Source: three-view drawing plus pictorial views. Frame: mm from the lowest corner of the part. A direction names the side the tool comes from. Give positions to 0.01 mm unless a question says otherwise; leave off trailing zeros. Order: outer loops, then holes, each group sorted by start corner. A loop starts at its lowest first (then second) coordinate and runs counter-clockwise, first axis right, second up. Notation, with made-up numbers: (-13.75, 50) -> (4.25, 50) arc R5 cw to (4.25, 55) -> close; hole circle Ø1 at (-6.75, 56.5). An arc over 180 degrees is marked (long way). Answer in a Markdown table with one row per item.
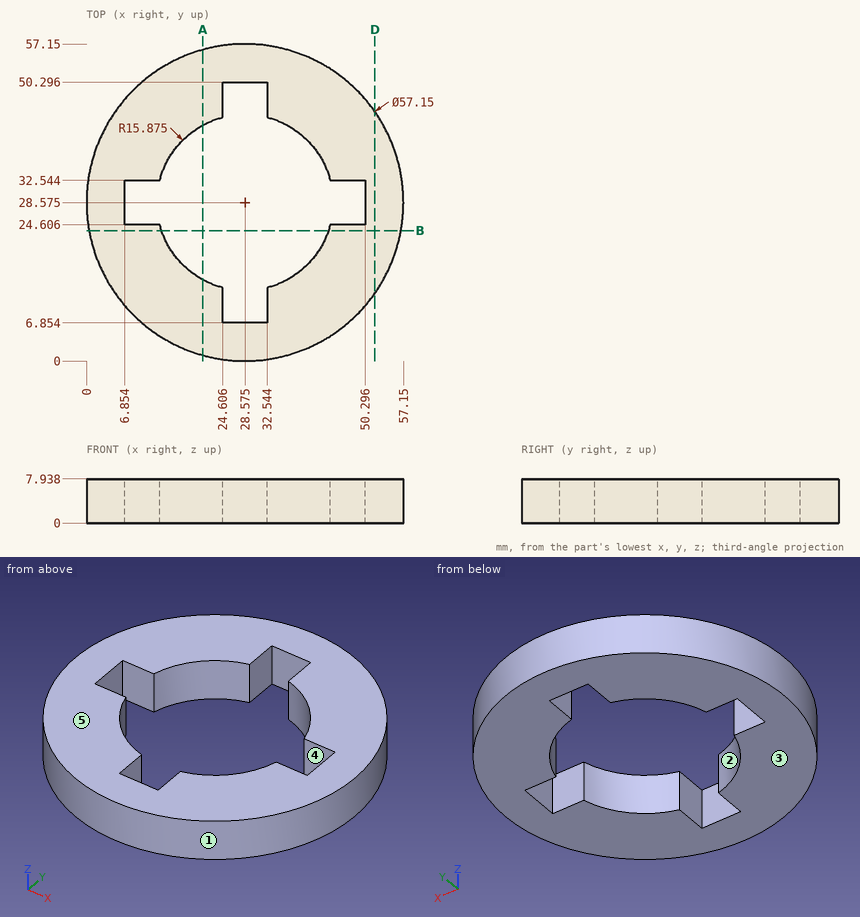
(1) Access query for the marked faces 4 and 5. Directions: +Z, -Z, +X, -X, +Y, -Y. A direction counts if a zero-diameter tool reaches every point of the face in a straight line with its end or side. Return the directions, or none.
A:
| item | result |
|---|---|
| face 4 | +Z, -Z |
| face 5 | +Z, +X, -X, +Y, -Y |
(2) Section query D-D (x = 52). Return the cut outline in (y, z).
A:
| item | result |
|---|---|
| outline | (12.21, 0) -> (44.94, 0) -> (44.94, 7.94) -> (12.21, 7.94) -> close |
(3) Section query B-B (y = 23.5). Return the cut outline in (x, z) (1 decimal).
A:
| item | result |
|---|---|
| outline | (0.5, 0) -> (13.5, 0) -> (13.5, 7.9) -> (0.5, 7.9) -> close; (43.6, 0) -> (56.7, 0) -> (56.7, 7.9) -> (43.6, 7.9) -> close |
(4) Ray query, probe 1 along X at (y, z) = (13, 6.75) (1 decimal); probe 2 along X at (y, z) = (37.5, 3) (1 decimal); probe 3 along Y at (x, z) = (27, 2.25) (1 decimal). Return the intervals inside material, ascending.
A:
| item | result |
|---|---|
| probe 1 | x = 4.6 to 24.6, 32.5 to 52.5 |
| probe 2 | x = 1.4 to 15.4, 41.7 to 55.7 |
| probe 3 | y = 0 to 6.9, 50.3 to 57.1 |
(5) Section query A-A (x = 21). Return the cut outline in (y, z).
A:
| item | result |
|---|---|
| outline | (1.02, 0) -> (14.62, 0) -> (14.62, 7.94) -> (1.02, 7.94) -> close; (42.53, 0) -> (56.13, 0) -> (56.13, 7.94) -> (42.53, 7.94) -> close |
(6) Pull-direction query (X, two-part tool) for the marked faces 1, 2 and 3; classes: +X half, -X half, draft (parallel to the pull), parting line (faces both ways), or undercut.
A:
| item | result |
|---|---|
| face 1 | parting line |
| face 2 | undercut |
| face 3 | draft |
(7) First-contact query: pin 1 Ø1 at (x, z) = (44, 3.5) entering from +Y; pin 2 Ø4 at (x, z) = (28, 3) entering from +Y; pin 3 Ø1.9 at (y, z) = (10.5, 4.5) entering from -X. Flat tips, straight axial feed; report the tip coordinate or a pass-through.
A:
| item | result |
|---|---|
| pin 1 | stops at y = 52.94 |
| pin 2 | stops at y = 57.15 |
| pin 3 | stops at x = 5.7 |
